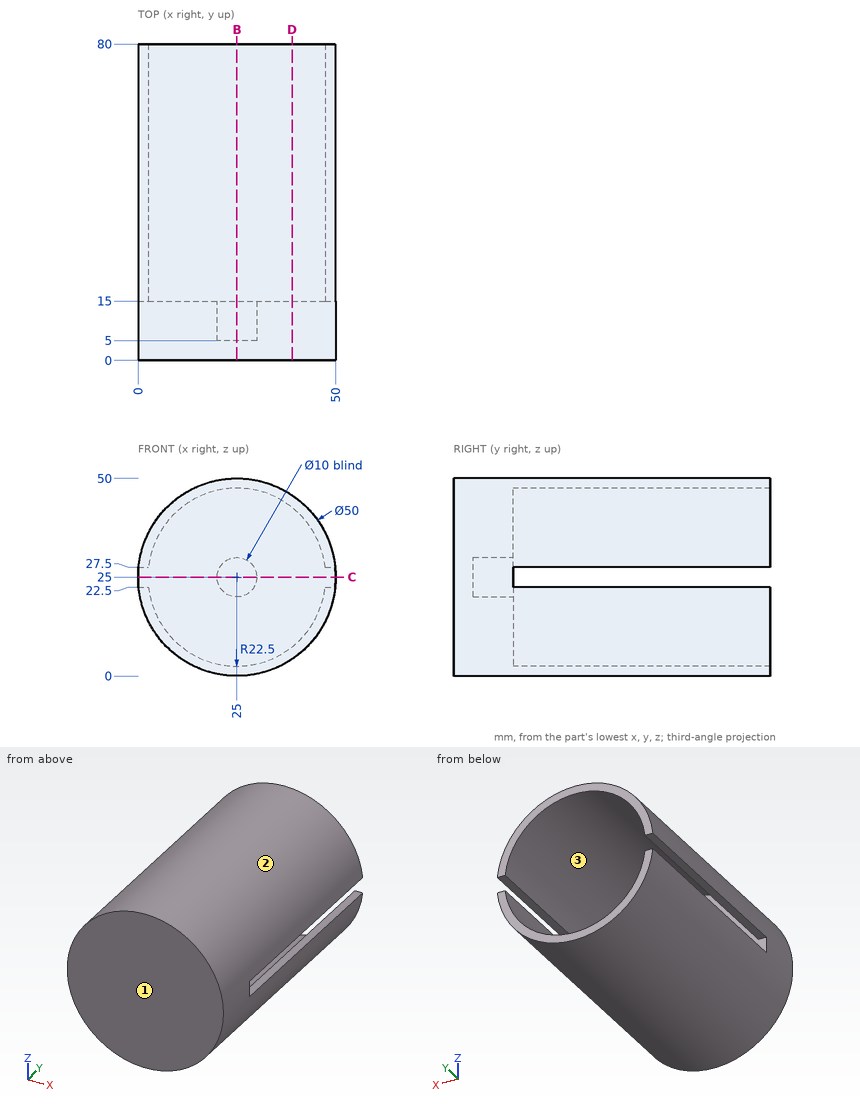
Geometry check sheet. Reference: drawing and pictorial views, mm from the part's lowest x, y, z. Coordinates: 2 decimals unless noted, no trailing zeros. Loops run counter-clockwise (first coordinate to the right, second up) from the corner with the lowest first, then second, coordinate; pieces in that order, holes last. Notation, with made-up numbers: (-4.5, -5.75) - (46.5, -5.75) arc R18 cw to (46.5, 23.25) - close; hole circle Ø9 at (46.25, 15). An arc over 180 degrees is marked (long way). Return JSON: item names as keys, results as strings.
1. Section check B-B, the plane x = 25. Record the boundary of the cut face in (y, z).
Established:
{"outline": "(0, 0) - (80, 0) - (80, 2.5) - (15, 2.5) - (15, 20) - (5, 20) - (5, 30) - (15, 30) - (15, 47.5) - (80, 47.5) - (80, 50) - (0, 50) - close"}
2. Mould release check, pull along X, two halves, no side actions. Record for the marked faces 1, 2 and 3: +X half, -X half, draft (parallel to the pull), parting line (faces both ways), or undercut.
Established:
{"face 1": "draft", "face 2": "parting line", "face 3": "undercut"}
3. Section check C-C, the plane z = 25. Record the boundary of the cut face in (x, y).
Established:
{"outline": "(0, 0) - (50, 0) - (50, 15) - (30, 15) - (30, 5) - (20, 5) - (20, 15) - (0, 15) - close"}
4. Section check D-D, the plane x = 39. Record the boundary of the cut face in (y, z), then the cut area to 3 significant figures.
Established:
{"outline": "(0, 4.29) - (80, 4.29) - (80, 7.39) - (15, 7.39) - (15, 42.61) - (80, 42.61) - (80, 45.71) - (0, 45.71) - close", "area": "1,020 mm2"}
5. Go/stop test with flat-tipped pins: pin 1 (6 mm diameter, centred on x = 18.5, z = 17.5, fed in from +Y); pin 2 (8 mm diameter, centred on y = 68.5, z = 35.5, fed in from +X); pin 3 (3 mm diameter, centred on x = 48.5, y = 55.5, fed in from -Z). Record where each tip stops, or that it passes through.
Established:
{"pin 1": "stops at y = 15", "pin 2": "stops at x = 49.14", "pin 3": "stops at z = 13.13"}
6. Thickness scan on L1, parallel to X at y = 13, z = 25; L2, parallel to Y at x = 35.5, z = 9.5. Record the ranges inside material, lowest first.
Established:
{"L1": "x = 0 to 20, 30 to 50", "L2": "y = 0 to 15"}
